Design review of the part built by this model. Coordinates are the model's own, in mm. Give positions to 0.01 mm unless a question says otherwise; leave off trailing zeros. Loops run counter-clockwise (first coordinate to the right, second up) from the corner with the lowest first, then second, coordinate; pieces in that order, holes last. Notation, with made-up numbers: M -32.5,30.5 L -5.5,30.5 A12 ccw -5.5,41.5 Z; hole C 14,14.5 d8. An arc over 180 degrees is marked long. Use a Markdown table: item, result. Add a question column.
(1) For probe 1 along X at (y, z) = (2.1, 22); probe 2 along Z at (x, y) = (59.5, 0.9); probe 3 along Z at (x, y) = (24.5, 2.9), list the stretches that pass through material, from the lowest coordinate up.
(2) Add section A-A, the plane z = -9. Give the boundary of the cut face in (x, y).
(3) Draft analysis for pull direction Z (two halves, no side actions). For faces 1 (the face through (63.927, 1.726, 56.246)), 2 (the face through (44, 2, 72.027)), 3 (the face through (116.646, 2, 23)), state which applies: pulls with the +Z half, pulls with the -Z half, needs draft (parallel to the pull), parting line crosses it, or undercut.
```python
from build123d import *

# Parameters (mm, degrees)
SKETCH1_W             = 143.5
SKETCH1_H             = 100
BOSS_EXTRUDE1_DEPTH   = 3.5
F_6_0MM_DOWEL_HOLE1_D = 6
F_6_0MM_DOWEL_HOLE2_D = 6
F_6_0MM_DOWEL_HOLE3_D = 6
F_6_0MM_DOWEL_HOLE4_D = 6
F_6_0MM_DOWEL_HOLE5_D = 6
F_6_0MM_DOWEL_HOLE6_D = 6


with BuildPart() as part:
    # Sketch1 → Boss-Extrude1 (new body)
    with BuildSketch(Plane(origin=(0, 0, 0), x_dir=(1, 0, 0), z_dir=(0, 1, 0))):
        with Locations((44.896177875, -22.027268619)):
            Rectangle(SKETCH1_W, SKETCH1_H)
    extrude(amount=BOSS_EXTRUDE1_DEPTH)

    # Ø6.0mm Dowel Hole1 (through all)
    with Locations(Plane(origin=(237.217905301, 3.5, -102.05218535), x_dir=(0, 0, 1), z_dir=(0, 1, 0))):
        with Locations((156.087532559, -175.318700205)):
            Hole(F_6_0MM_DOWEL_HOLE1_D / 2)

    # Ø6.0mm Dowel Hole2 (through all)
    with Locations(Plane(origin=(237.217905301, 3.5, -102.05218535), x_dir=(0, 0, 1), z_dir=(0, 1, 0))):
        with Locations((123.097877986, -175.280990501)):
            Hole(F_6_0MM_DOWEL_HOLE2_D / 2)

    # Ø6.0mm Dowel Hole3 (through all)
    with Locations(Plane(origin=(237.217905301, 3.5, -102.05218535), x_dir=(0, 0, 1), z_dir=(0, 1, 0))):
        with Locations((123.026211567, -213.535463753)):
            Hole(F_6_0MM_DOWEL_HOLE3_D / 2)

    # Ø6.0mm Dowel Hole4 (through all)
    with Locations(Plane(origin=(237.217905301, 3.5, -102.05218535), x_dir=(0, 0, 1), z_dir=(0, 1, 0))):
        with Locations((155.91154644, -213.495641578)):
            Hole(F_6_0MM_DOWEL_HOLE4_D / 2)

    # Ø6.0mm Dowel Hole5 (through all)
    with Locations(Plane(origin=(237.217905301, 3.5, -102.05218535), x_dir=(0, 0, 1), z_dir=(0, 1, 0))):
        with Locations((91.479185985, -213.996610116)):
            Hole(F_6_0MM_DOWEL_HOLE5_D / 2)

    # Ø6.0mm Dowel Hole6 (through all)
    with Locations(Plane(origin=(237.217905301, 3.5, -102.05218535), x_dir=(0, 0, 1), z_dir=(0, 1, 0))):
        with Locations((91.901828901, -175.454462016)):
            Hole(F_6_0MM_DOWEL_HOLE6_D / 2)


solid = part.part
```
Established:
| question | item | result |
|---|---|---|
| 1 | probe 1 | -26.85 to 20.86, 26.5 to 59.09, 64.78 to 116.65 |
| 1 | probe 2 | -27.97 to -12.12, -8.18 to 19.3, 22.8 to 52.23, 55.84 to 72.03 |
| 1 | probe 3 | -27.97 to -13.29, -7.86 to 18.09, 23.86 to 50.96, 56.76 to 72.03 |
| 2 | outline | M -26.85,0 L 20.67,0 L 20.67,3.5 L -26.85,3.5 Z; M 25.78,0 L 58.99,0 L 58.99,3.5 L 25.78,3.5 Z; M 64.53,0 L 116.65,0 L 116.65,3.5 L 64.53,3.5 Z |
| 3 | face 1 | undercut |
| 3 | face 2 | pulls with the +Z half |
| 3 | face 3 | needs draft |
